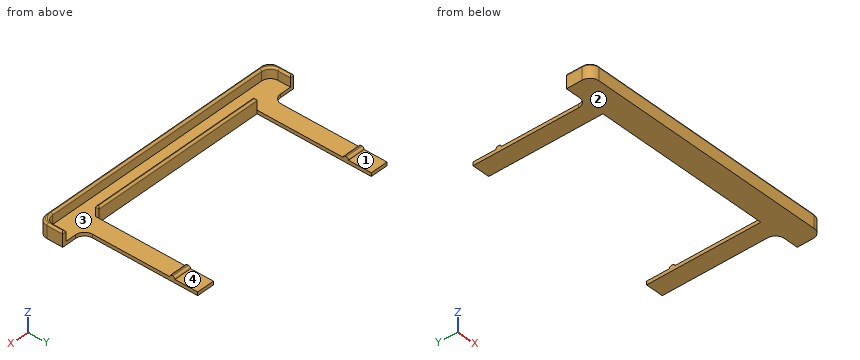
```python
from build123d import *

# Parameters (mm, degrees)
F2_W     = 10
F2_H     = 65
F2_W_2   = 11.25
F2_H_2   = 12
F2_W_3   = 100.5
F2_H_3   = 2
F2_W_4   = 2
F2_H_4   = 10
F3_DEPTH = 2
F4_DEPTH = 8
F5_R     = 5
F6_R     = 0.99999
F7_W     = 10
F7_H     = 3
F8_DEPTH = 1.2
F9_R     = 1.19999


# Not quite as in the source:
# - a fillet or chamfer is up to 0.001 mm smaller than in the source, because OpenCascade refuses the exact size


with BuildPart() as f3:
    # F2 (on Top) → F3 (new body)
    with BuildSketch(Plane.XY):
        with Locations((-47.7500067828, 32.5)):
            Rectangle(F2_W, F2_H)
        Polygon((-42.7500067828, 0), (-52.7500067828, 0), (-52.7500067828, -12), (-42.7500067828, -12), (-42.7500067828, -2), align=None)
        with Locations((-58.3750067828, -6)):
            Rectangle(F2_W_2, F2_H_2)
        with Locations((7.4999932172, -1)):
            Rectangle(F2_W_3, F2_H_3)
        Polygon((-42.7500067828, -12), (-52.7500067828, -12), (-64.0000067828, -12), (-66.0000067828, -12), (-66.0000067828, -14), (80.9999932172, -14), (80.9999932172, -12), (78.9999932172, -12), (67.7499932172, -12), (57.7499932172, -12), align=None)
        with Locations((-65.0000067828, -6)):
            Rectangle(F2_W_4, F2_H_2)
        with Locations((62.7499932172, 32.5)):
            Rectangle(F2_W, F2_H)
        Polygon((67.7499932172, 0), (57.7499932172, 0), (57.7499932172, -2), (57.7499932172, -12), (67.7499932172, -12), align=None)
        with Locations((73.3749932172, -6)):
            Rectangle(F2_W_2, F2_H_2)
        with Locations((79.9999932172, -6)):
            Rectangle(F2_W_4, F2_H_2)
        with Locations((7.4999932172, -7)):
            Rectangle(F2_W_3, F2_H_4)
    extrude(amount=F3_DEPTH)

    # F2 (on Top) → F4 (join)
    with BuildSketch(Plane.XY):
        with Locations((-65.0000067828, -6)):
            Rectangle(F2_W_4, F2_H_2)
        Polygon((-42.7500067828, -12), (-52.7500067828, -12), (-64.0000067828, -12), (-66.0000067828, -12), (-66.0000067828, -14), (80.9999932172, -14), (80.9999932172, -12), (78.9999932172, -12), (67.7499932172, -12), (57.7499932172, -12), align=None)
        with Locations((79.9999932172, -6)):
            Rectangle(F2_W_4, F2_H_2)
        with Locations((7.4999932172, -1)):
            Rectangle(F2_W_3, F2_H_3)
    extrude(amount=F4_DEPTH)

    # F5
    f5_edges = [f3.edges().sort_by_distance(p)[0] for p in [
        (-66.000007, -14, 4),
        (80.999993, -14, 4),
        (-64.000007, -12, 5),
        (78.999993, -12, 5),
        (67.749993, 0, 1),
        (-52.750007, 0, 1),
    ]]
    fillet(f5_edges, radius=F5_R)

    # F6 (radius 1 in the source; OpenCascade refuses exactly that, so slightly less here)
    f6_edges = [f3.edges().sort_by_distance(p)[0] for p in [
        (7.499993, -14, 8),
        (7.499993, -12, 8),
        (79.999993, 0, 8),
        (-65.000007, 0, 8),
        (7.499993, -2, 8),
        (7.499993, 0, 8),
        (57.749993, -1, 8),
        (-42.750007, -1, 8),
    ]]
    fillet(f6_edges, radius=F6_R)

    # F7 (on face) → F8 (join)
    with BuildSketch(Plane.XY.offset(2)):
        with Locations((-47.7500067828, 50.5)):
            Rectangle(F7_W, F7_H)
        with Locations((62.7499932172, 50.5)):
            Rectangle(F7_W, F7_H)
    extrude(amount=F8_DEPTH)

    # F9 (radius 1.2 in the source; OpenCascade refuses exactly that, so slightly less here)
    f9_edges = [f3.edges().sort_by_distance(p)[0] for p in [
        (-47.750007, 49, 3.2),
        (-47.750007, 52, 3.2),
        (62.749993, 49, 3.2),
        (62.749993, 52, 3.2),
    ]]
    fillet(f9_edges, radius=F9_R)


solid = f3.part
```
Here's how the part is built. I have some questions about the finished solid (model axes, mm). Face numbers are marked on the shaded views. A direction names the side the tool comes from. Coordinates: 2 decimals unless noted, no trailing zeros. Write each loop counter-clockwise with the first axis right and the second up, starting at its lowest first coordinate (ties: lowest second). Pieces come first, ordered by that corner, then holes. Notation, with made-up numbers: (49, 26) -> (66, 26) arc R21 ccw to (66, 43) -> close; hole circle Ø4 at (15.25, 20.25). An arc over 180 degrees is marked (long way). Use a Markdown table: item, result. Add a question column.
(1) I'm going to push flat-ended pins straight in: P1, Ø3.5, axis at x = 77.5, z = 3.5, coming from the +Y side; P2, Ø3.5, axis at y = 35.5, z = 2, coming from the -X side; P3, Ø0.7, axis at x = 64, y = 50.5, coming from the +Z side. Where does each tip first touch, or does it pass through?
(2) If we section it at A-A, the plane y = 59: Write out the boundary of the cut face in (x, z), and give its area (3 significant figures).
(3) We'd pull the mould along Y, two halves only. Please class the marked faces 3 and 4: +Y half, -Y half, draft (parallel to the pull), parting line (faces both ways), or undercut.
(4) If we section it at B-B, the plane z = 5.25: Write out the boundary of the cut face in (x, y), and give its area (3 significant figures).
(5) For the marked faces 1 and 2, which set-ups out of +Z, -Z, +X, -X, +Y, -Y let a thin tool reach every point of the face, with its end or its side?
(6) Please list where these lines run through material, in increasing order: line 1 (X direction, y = -1, z = 6.75); line 2 (Y direction, x = 51, z = 5.25); line 3 (X direction, y = 51.5, z = 2.25).
Outcome:
| question | item | result |
|---|---|---|
| 1 | P1 | stops at y = 0 |
| 1 | P2 | stops at x = -52.75 |
| 1 | P3 | stops at z = 3.2 |
| 2 | outline | (-52.75, 0) -> (-42.75, 0) -> (-42.75, 2) -> (-52.75, 2) -> close; (57.75, 0) -> (67.75, 0) -> (67.75, 2) -> (57.75, 2) -> close |
| 2 | area | 40.0 mm^2 |
| 3 | face 3 | undercut |
| 3 | face 4 | draft |
| 4 | outline | (-66, -9) arc R5 ccw to (-61, -14) -> (76, -14) arc R5 ccw to (81, -9) -> (81, 0) -> (79, 0) -> (79, -7) arc R5 cw to (74, -12) -> (-59, -12) arc R5 cw to (-64, -7) -> (-64, 0) -> (-66, 0) -> close; (-42.75, -2) -> (57.75, -2) -> (57.75, 0) -> (-42.75, 0) -> close |
| 4 | area | 543 mm^2 |
| 5 | face 1 | +Z, +X, -X, +Y |
| 5 | face 2 | -Z, +X, -X, +Y, -Y |
| 6 | line 1 | x = -66 to -64, -42.75 to 57.75, 79 to 81 |
| 6 | line 2 | y = -14 to -12, -2 to 0 |
| 6 | line 3 | x = -52.75 to -42.75, 57.75 to 67.75 |
